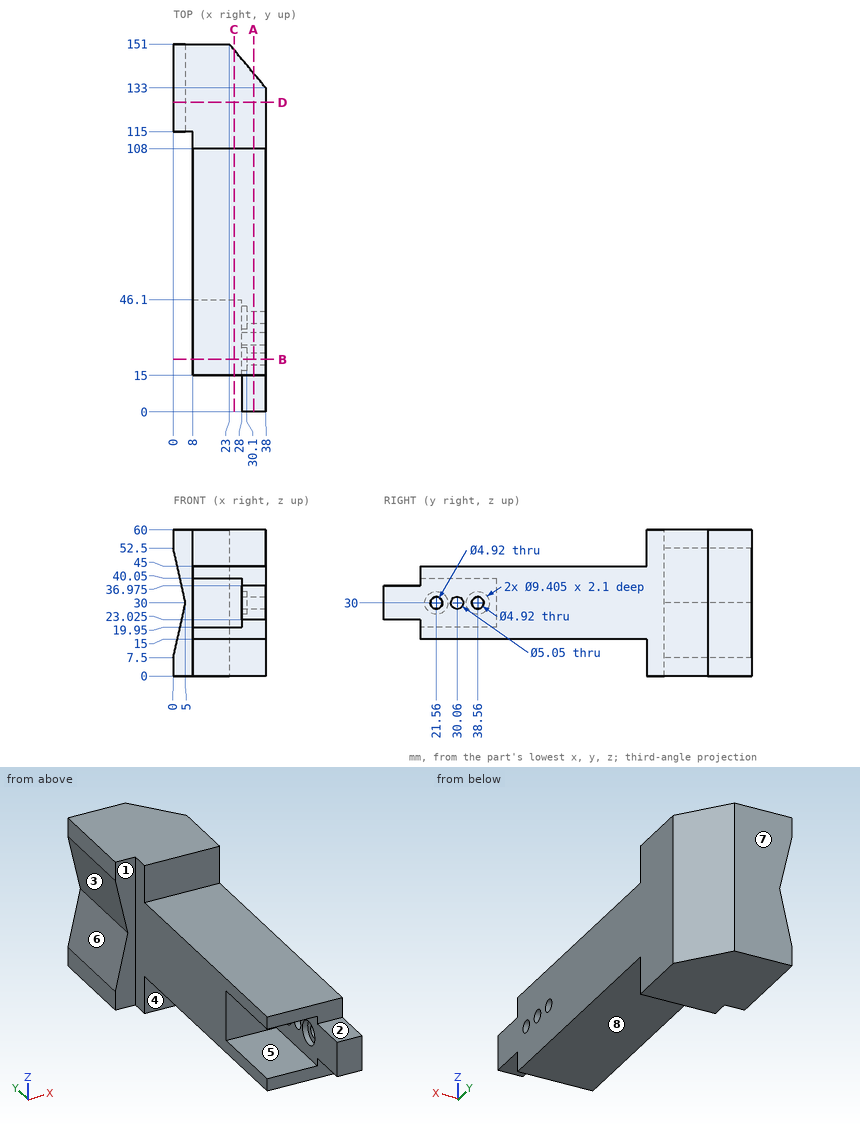
Can you work these out from the drawing? Everything is in mm from the part's minimum corner. A direction names the side the tool comes from. Give positions to 0.01 mm unless a question says otherwise; leave off trailing zeros. Loops run counter-clockwise (first coordinate to the right, second up) from the corner with the lowest first, then second, coordinate; pieces in that order, holes last. Notation, with made-up numbers: (74, 52.5) -> (88, 52.5) arc R27 ccw to (88, 81.5) -> close; hole circle Ø5 at (30, -3). An arc over 180 degrees is marked (long way). Return JSON: item names as keys, results as strings.
Q1. I want a section at B-B, the plane y = 21.56. List the corners of the cut face in (x, z) for me, then the cut area to 3 significant figures.
Checks:
{"outline": "(8, 15) -> (38, 15) -> (38, 27.54) -> (30.1, 27.54) -> (30.1, 25.3) -> (28, 25.3) -> (28, 19.95) -> (8, 19.95) -> close; (8, 40.05) -> (28, 40.05) -> (28, 34.7) -> (30.1, 34.7) -> (30.1, 32.46) -> (38, 32.46) -> (38, 45) -> (8, 45) -> close", "area": "439 mm2"}
Q2. I want a section at D-D, the plane y = 127. List the corners of the cut face in (x, z) for me, then the cut area to 3 significant figures.
Checks:
{"outline": "(0, 0) -> (38, 0) -> (38, 60) -> (0, 60) -> (0, 52.5) -> (5, 30) -> (0, 7.5) -> close", "area": "2,170 mm2"}
Q3. I want a section at A-A, the plane x = 33. List the corners of the cut face in (y, z) for me (3 decimals).
Checks:
{"outline": "(0, 23.025) -> (15, 23.025) -> (15, 15) -> (108, 15) -> (108, 0) -> (139, 0) -> (139, 60) -> (108, 60) -> (108, 45) -> (15, 45) -> (15, 36.975) -> (0, 36.975) -> close; hole circle Ø4.92 at (21.56, 30); hole circle Ø5.05 at (30.06, 30); hole circle Ø4.92 at (38.56, 30)"}
Q4. I want a section at C-C, the plane x = 25. List the corners of the cut face in (y, z) for me, then the cut area to 3 significant figures.
Checks:
{"outline": "(15, 15) -> (108, 15) -> (108, 0) -> (148.6, 0) -> (148.6, 60) -> (108, 60) -> (108, 45) -> (15, 45) -> (15, 40.05) -> (46.1, 40.05) -> (46.1, 19.95) -> (15, 19.95) -> close", "area": "4,600 mm2"}
Q5. On a 3-axis mill with a long thin cutter (end or side, diameter ignored), from which of +Z, -Z, +X, -X, +Y, -Y can I reach the whole of each face in a straight line? I mean the marked faces 1, 2, 3 and 4. Say none if no direction works.
Checks:
{"face 1": "+Z, -Z, -X, -Y", "face 2": "+Z, +X, -X, -Y", "face 3": "-X, +Y, -Y", "face 4": "-Z, +X, -X, -Y"}
Q6. We'd pull the mould along Z, two halves only. Please class the marked faces 5, 6, 7 and 8: released by +Z, released by -Z, zero draft, split by the parting line, or undercut.
Checks:
{"face 5": "undercut", "face 6": "undercut", "face 7": "zero draft", "face 8": "released by -Z"}
Q7. For pin 1 Ø22 at (x, y) = (20.5, 37) entering from +Z; pin 2 Ø8 at (x, y) = (12, 89) entering from -Z; pin 3 Ø4.5 at (y, z) = (30.06, 30) entering from -X; pin 4 Ø12 at (x, z) = (27.5, 56) entering from -Y, each with a flat end and sliding along its axis, tell me the tip position at first contact or that it passes through.
Checks:
{"pin 1": "stops at z = 45", "pin 2": "stops at z = 15", "pin 3": "passes through", "pin 4": "stops at y = 108"}
Q8. I need wall thicknesses on probe 1 along Y at (x, z) = (31, 30.5) (3 decimals); probe 2 along Z at (x, y) = (35, 30); probe 3 along Y at (x, z) = (32.75, 30) (3 decimals). Which ranges of each line are inside material? Lowest first, please.
Checks:
{"probe 1": "y = 0 to 19.151, 23.969 to 27.585, 32.535 to 36.151, 40.969 to 141.4", "probe 2": "z = 15 to 27.48, 32.52 to 45", "probe 3": "y = 0 to 19.1, 24.02 to 27.535, 32.585 to 36.1, 41.02 to 139.3"}
